from build123d import *

# Parameters (mm, degrees)
SALIENTE_EXTRUIR1_DEPTH = 6
CROQUIS2_R              = 8.1
SALIENTE_EXTRUIR2_DEPTH = 3
REDONDEO1_R             = 2
CROQUIS3_R              = 5
SALIENTE_EXTRUIR3_DEPTH = 500


with BuildPart() as part:
    # Croquis1 → Saliente-Extruir1 (new body)
    with BuildSketch(Plane(origin=(0, 0, 0), x_dir=(1, 0, 0), z_dir=(0, 1, 0))):
        Polygon((4.907477288, -8.5), (9.814954576, 0), (4.907477288, 8.5), (-4.907477288, 8.5), (-9.814954576, 0), (-4.907477288, -8.5), align=None)
    extrude(amount=SALIENTE_EXTRUIR1_DEPTH)

    # Croquis2 → Saliente-Extruir2 (add)
    with BuildSketch(Plane.XZ):
        with Locations(Location((0, 0, 0), (0, 0, 270))):
            Circle(CROQUIS2_R)
    extrude(amount=SALIENTE_EXTRUIR2_DEPTH)

    # Redondeo1
    redondeo1_edges = [part.edges().sort_by_distance(p)[0] for p in [
        (0, -3, 8.1),
    ]]
    fillet(redondeo1_edges, radius=REDONDEO1_R)

    # Croquis3 → Saliente-Extruir3 (add)
    with BuildSketch(Plane(origin=(0, 6, 0), x_dir=(1, 0, 0), z_dir=(0, 1, 0))):
        with Locations(Location((0, 0, 0), (0, 0, 270))):
            Circle(CROQUIS3_R)
    extrude(amount=SALIENTE_EXTRUIR3_DEPTH)


solid = part.part
Input: part model. Units: mm. Frame: model coordinates. A direction names the side the tool comes from. Give positions to 0.01 mm unless a question says otherwise; leave off trailing zeros. Order: outer loops, then holes, each group sorted by start corner. A loop starts at its lowest first (then second) coordinate and runs counter-clockwise, first axis right, second up. Notation, with made-up numbers: M -22.5,51.25 L 6.5,51.25 A20 ccw 6.5,79.25 Z; hole C -34.5,18 d7. An arc over 180 degrees is marked long. Answer as a JSON object with one key per item and string values.
1. Cut plane B-B, the plane y = 32. Output: boundary loops of the cut face in (x, z).
Result sheet:
{"outline": "C 0,0 d10"}
2. Ray query, line 1 (Z direction, x = -0.25, y = 348); line 2 (Y direction, x = 5, z = -2); line 3 (X direction, y = 178, z = 1.25). Return the intervals inside material, ascending. Write a range as [from, to].
Result sheet:
{"line 1": "[-4.99, 4.99]", "line 2": "[-3, 6]", "line 3": "[-4.84, 4.84]"}
3. Reachability of faces 1 (the flat face through (0, 506, 0)), 2 (the cylindrical face through (-4.88, 252.5, -1.08)), 3 (the flat face through (8, 0, 2.5)) from +Z, -Z, +X, -X, +Y, -Y: full face, straight path, thin tool, end or side. Return the list, or none.
Result sheet:
{"face 1": "+Z, -Z, +X, -X, +Y", "face 2": "+Y", "face 3": "-Y"}
4. First-contact query: P1, Ø3, axis at x = -6.5, z = -5.5, coming from the -Y side; P2, Ø4, axis at y = 421, z = -5.5, coming from the +X side; P3, Ø5, axis at x = 7, y = 244, coming from the +Z side. Flat tips, straight axial feed; report the tip coordinate or a pass-through.
Result sheet:
{"P1": "y = -2.78", "P2": "x = 3.57", "P3": "z = 2.18"}
5. Cut plane A-A, the plane x = 0. Output: boundary loops of the cut face in (y, z), and give its area (3 significant figures).
Result sheet:
{"outline": "M -3,-6.1 A2 ccw -1,-8.1 L 0,-8.1 L 0,-8.5 L 6,-8.5 L 6,-5 L 506,-5 L 506,5 L 6,5 L 6,8.5 L 0,8.5 L 0,8.1 L -1,8.1 A2 ccw -3,6.1 Z", "area": "5,150 mm²"}
